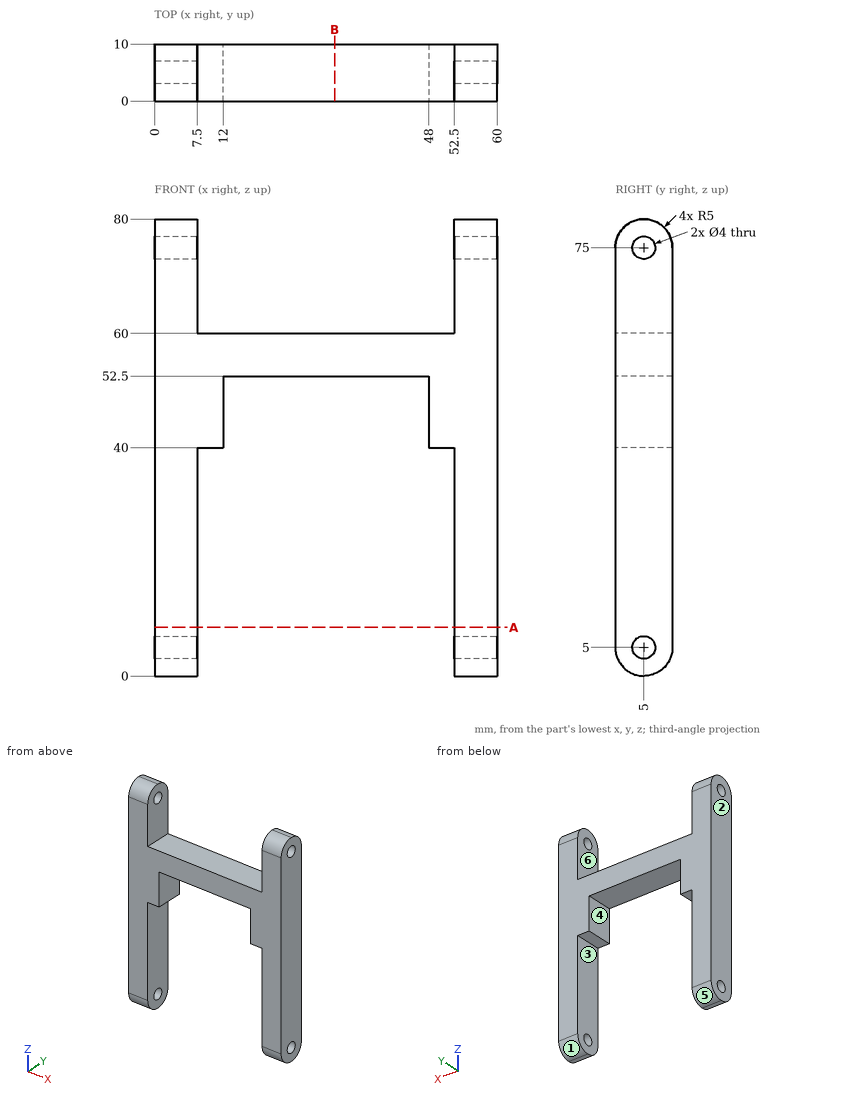
Part print with two shaded views. Sizes in mm from the minimum x, y, z corner. A direction names the side the tool comes from. Give positions to 0.01 mm unless a question says otherwise; leave off trailing zeros. Order: outer loops, then holes, each group sorted by start corner. A loop starts at its lowest first (then second) coordinate and runs counter-clockwise, first axis right, second up.
(1) Flat gauge pins, fed straight in: pin 1 (5 mm diameter, centred on x = 27, y = 4.5, fed in from -Z); pin 2 (5 mm diameter, centred on x = 36.5, y = 5.5, fed in from +Z); pin 3 (3.5 mm diameter, centred on x = 9.5, y = 7.5, fed in from -Z). Where does each tip first touch, or does it go through?
(2) Saw through at A-A, the plane z = 8.5. Give the cut face in (x, y), then the cut area to 3 significant figures.
(3) Tool access for the marked faces 4, 5 and 6: list every direction of +Z, -Z, +X, -X, +Y, -Y with a clear straight run to the whole face (end or side of a thin tool).
(4) Mould opens along X. For the marked faces 1, 2 and 3 say: released by +X, released by -X, zero draft, split by the parting line, or undercut.
(5) Saw through at B-B, the plane x = 31.5. Give the cut face in (y, z), then the cut area to 3 significant figures.
(6) Drill centre lines: L1, parallel to X at y = 3.25, z = 43.5; L2, parallel to Y at x = 6, z = 75; L3, parallel to X at y = 7, z = 74. Where is each one in solid material? Low to high.
Results found:
1. pin 1: stops at z = 52.5
1. pin 2: stops at z = 60
1. pin 3: stops at z = 40
2. outline: (0, 0) - (7.5, 0) - (7.5, 10) - (0, 10) - close; (52.5, 0) - (60, 0) - (60, 10) - (52.5, 10) - close
2. area: 150 mm2
3. face 4: -Z, +Y, -Y
3. face 5: -Z, +X, -X, +Y
3. face 6: +Z, +Y, -Y
4. face 1: zero draft
4. face 2: released by -X
4. face 3: undercut
5. outline: (0, 52.5) - (10, 52.5) - (10, 60) - (0, 60) - close
5. area: 75.0 mm2
6. L1: x = 0 to 12, 48 to 60
6. L2: y = 0 to 3, 7 to 10
6. L3: x = 0 to 7.5, 52.5 to 60
